Geometry: see drawing. Coordinates: mm, zero at the bounding-box minimum. Give positions to 0.01 mm unless a question says otherwise; leave off trailing zeros. Write each loop counter-clockwise with the first axis right and the second up, starting at its lowest first coordinate (ties: lowest second). Pieces come first, ordered by that corner, then holes. Notation, with made-up numbers: (8.5, -38.75) - (24.5, -38.75) arc R16 ccw to (24.5, -17.75) - close; hole circle Ø4 at (-10.75, 16.5). An arc over 180 degrees is marked (long way). Answer as CSV lines item,"result". Start each with the question number.
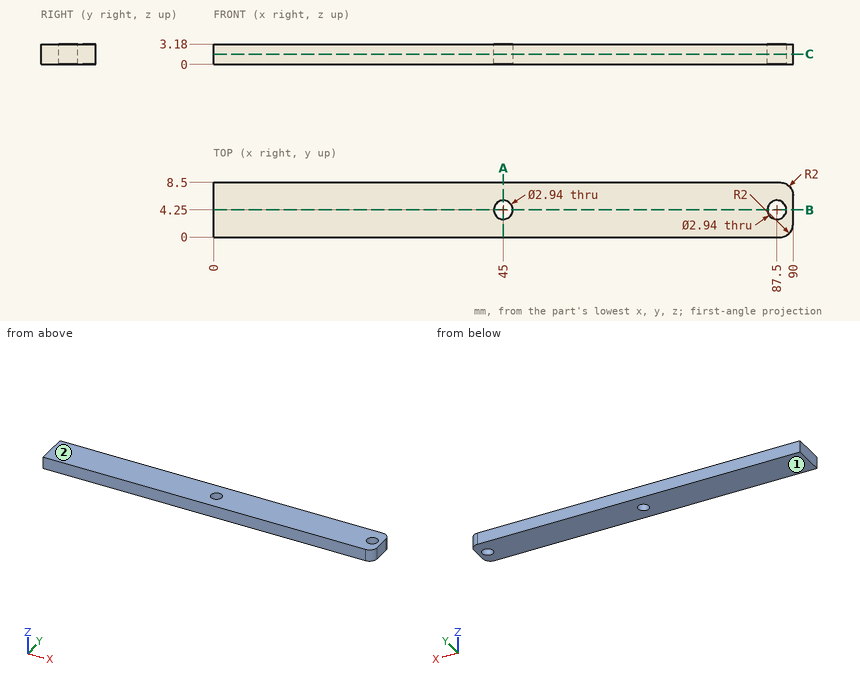
1) Cut plane C-C on z = 1.6. Output: boundary loops of the cut face in (x, y).
2) Cut plane A-A on x = 45. Output: boundary loops of the cut face in (y, z), and give its area (3 significant figures).
3) Pull-direction query (Z, two-part tool) for the marked faces 1 and 2; classes: +Z half, -Z half, draft (parallel to the pull), parting line (faces both ways), or undercut.
4) Contact query for a flat-ended pin moving along its axis: P1, Ø1.5, axis at y = 4.5, z = 3, coming from the -X side. Output: stop coordinate, or through.
5) Cut plane B-B on y = 4.25. Output: boundary loops of the cut face in (x, z).
6) Material intervals for line 1 (Y direction, x = 87.5, z = 1.3); line 2 (X direction, y = 3.5, z = 2.5); line 3 (X direction, y = 1.75, z = 2.6), sorted ascending. Write a range as from..to.
Numbers:
1,outline,"(0, 0) - (88, 0) arc R2 ccw to (90, 2) - (90, 6.5) arc R2 ccw to (88, 8.5) - (0, 8.5) - close; hole circle Ø2.94 at (45, 4.25); hole circle Ø2.94 at (87.5, 4.25)"
2,outline,"(0, 0) - (2.78, 0) - (2.78, 3.18) - (0, 3.18) - close; (5.72, 0) - (8.5, 0) - (8.5, 3.18) - (5.72, 3.18) - close"
2,area,"17.7 mm²"
3,face 1,"-Z half"
3,face 2,"+Z half"
4,P1,"stops at x = 0"
5,outline,"(0, 0) - (43.53, 0) - (43.53, 3.18) - (0, 3.18) - close; (46.47, 0) - (86.03, 0) - (86.03, 3.18) - (46.47, 3.18) - close; (88.97, 0) - (90, 0) - (90, 3.18) - (88.97, 3.18) - close"
6,line 1,"y = 0..2.78, 5.72..8.5"
6,line 2,"x = 0..43.74, 46.26..86.24, 88.76..90"
6,line 3,"x = 0..89.98"
